Design review of the part built by this model. Coordinates are the model's own, in mm. A direction names the side the tool comes from. Give positions to 0.01 mm unless a question says otherwise; leave off trailing zeros. Loops run counter-clockwise (first coordinate to the right, second up) from the corner with the lowest first, then second, coordinate; pieces in that order, holes last. Notation, with made-up numbers: M 69.5,4.5 L 93.5,4.5 A19 cw 93.5,10.5 Z; hole C 23.5,46 d4. An arc over 180 degrees is marked long. Answer as CSV lines item,"result".
```python
from build123d import *

# Parameters (mm, degrees)
SKETCH_R     = 6
PAD_DEPTH    = 1
PAD001_DEPTH = 20
FILLET_R     = 1
CHAMFER_SIZE = 0.5


with BuildPart() as part:
    # Sketch → Pad (new body)
    with BuildSketch(Plane.XY):
        Circle(SKETCH_R)
        with BuildLine():
            ThreePointArc((-1.24499, 1.3), (0, -1.8), (1.24499, 1.3))
            Line((-1.24499, 1.3), (1.24499, 1.3))
        make_face(mode=Mode.SUBTRACT)
    extrude(amount=-PAD_DEPTH)

    # Sketch001 → Pad001 (join)
    with BuildSketch(Plane.XY):
        Polygon((-5.196152, 3), (5.196152, 3), (0, -6), align=None)
        with BuildLine():
            ThreePointArc((-1.24499, 1.3), (0, -1.8), (1.24499, 1.3))
            Line((-1.24499, 1.3), (1.24499, 1.3))
        make_face(mode=Mode.SUBTRACT)
    extrude(amount=PAD001_DEPTH)

    # Fillet
    fillet_edges = [part.edges().sort_by_distance(p)[0] for p in [
        (0, -6, 10),
        (5.196152, 3, 10),
        (-5.196152, 3, 10),
    ]]
    fillet(fillet_edges, radius=FILLET_R)

    # Chamfer
    chamfer_edges = [part.edges().sort_by_distance(p)[0] for p in [
        (-2.598076, -1.5, 20),
    ]]
    chamfer(chamfer_edges, length=CHAMFER_SIZE)


solid = part.part
```
1. For faces 1 (the flat face through (-2.6, -1.5, 9.6)), 2 (the cylindrical face through (-4.323, 2.513, 9.886)), 3 (the flat face through (2.6, -1.5, 9.6)), list the 3-axis set-ups (+Z, -Z, +X, -X, +Y, -Y) from which the entire face can be reached by the end or side of a thin tool; tool diameter is ignored.
Answer block:
face 1,"+Z, -X, -Y"
face 2,"+Z, -X"
face 3,"+Z, +X, -Y"
2. For P1, Ø5, axis at y = -1, z = 14, coming from the +X side; P2, Ø1, axis at y = 0.5, z = 5, coming from the +X side; P3, Ø1, axis at x = -3, z = 4, coming from the +Y side, all flat-tipped, find the tip position at first contact; note any pin that passes through.
Answer block:
P1,"x = 4.33"
P2,"x = 4.04"
P3,"y = 3"
3. The part is to be moulded in two halves that separate along X. For faces 4 (the cylindrical face through (0, -5, 10)), 5 (the cylindrical face through (-0.06, -1.8, 9.35)), 6 (the flat face through (0, 1.3, 9)), 7 (the flat face through (-2.36, -1.419, 19.746)), say which applies: pulls with the +X half, pulls with the -X half, needs draft (parallel to the pull), parting line crosses it, or undercut.
Answer block:
face 4,"parting line crosses it"
face 5,"undercut"
face 6,"undercut"
face 7,"pulls with the -X half"
4. To check wall thickness, follow L1, parallel to X at y = 0, z = 3.5; L2, parallel to Z at x = -0.75, y = 4.75; L3, parallel to Y at x = 0.75, z = 16. State the ranges of each line that lie inside material, in increasing order. Write a range as [from, to].
Answer block:
L1,"[-3.46, -1.8], [1.8, 3.46]"
L2,"[-1, 0]"
L3,"[-4.66, -1.64], [1.3, 3]"
5. We need section B-B, the plane z = 8.5. Write out the cut boundary in (x, y) (3 decimals).
Answer block:
outline,"M -4.33,1.5 L -0.866,-4.5 A1 ccw 0.866,-4.5 L 4.33,1.5 A1 ccw 3.464,3 L -3.464,3 A1 ccw Z; hole M -1.245,1.3 A1.8 ccw long 1.245,1.3 Z"
6. We need section C-C, the plane y = -0.25. Write out the cut boundary in (x, z), plus the area to 3 significant figures.
Answer block:
outline,"M -5.99,-1 L -1.78,-1 L -1.78,20 L -2.74,20 L -3.32,19.5 L -3.32,0 L -5.99,0 Z; M 1.78,-1 L 5.99,-1 L 5.99,0 L 3.32,0 L 3.32,19.5 L 2.74,20 L 1.78,20 Z"
area,"69.6 mm²"
7. We need section D-D, the plane x = 2.25. Write out the cut boundary in (y, z).
Answer block:
outline,"M -5.56,-1 L 5.56,-1 L 5.56,0 L 3,0 L 3,19.5 L 2.5,20 L -1.1,20 L -2.1,19.5 L -2.1,0 L -5.56,0 Z"
8. We need section A-A, the plane x = 0. Write out the cut boundary in (y, z), plus the area to 3 significant figures.
Answer block:
outline,"M -6,-1 L -1.8,-1 L -1.8,20 L -4.5,20 L -5,19.5 L -5,0 L -6,0 Z; M 1.3,-1 L 6,-1 L 6,0 L 3,0 L 3,19.5 L 2.5,20 L 1.3,20 Z"
area,"107 mm²"
